Source: CAD feature listing. Evaluate the final solid. Frame: model axes, mm. Face numbers are marked on the shaded views. Coordinates: 2 decimals unless noted, no trailing zeros. Write each loop counter-clockwise with the first axis right and the second up, starting at its lowest first coordinate (ties: lowest second). Pieces come first, ordered by that corner, then holes. Notation, with made-up numbers: M 58.5,17.25 L 91.5,17.25 A32 cw 91.5,46.25 Z; hole C -23.5,-17.75 d6. An arc over 180 degrees is marked long. Write item = value, one per line. Start each with the question number.
1. Section query C-C (z = 4). Output: boundary loops of the cut face in (x, y), then the cut area to 3 significant figures.
2. Section query A-A (z = 11.5). Output: boundary loops of the cut face in (x, y), then the cut area to 3 significant figures.
3. Line query: line 1 along Y through (x, z) = (3.75, 12.5); line 2 along Z through (x, y) = (4.25, 1.75); line 3 along Y through (x, z) = (-6.5, -5). Output: solid intervals per line, ascending.
4. Pin query (flat end, axial travel): pin 1 Ø9 at (x, z) = (-2, 5) entering from -Y; pin 2 Ø4 at (x, y) = (4, -4) entering from +Z. Return the tip coordinate at first contact, or that it passes through.
5. Section query D-D (y = -2.5). Output: boundary loops of the cut face in (x, z).
6. Section query B-B (x = -2). Output: boundary loops of the cut face in (y, z), then the cut area to 3 significant figures.
7. Pull-direction query (Y, two-part tool) for the marked faces 1 and 2; classes: pulls with the +Y half, pulls with the -Y half, needs draft (parallel to the pull), parting line crosses it, or undercut.
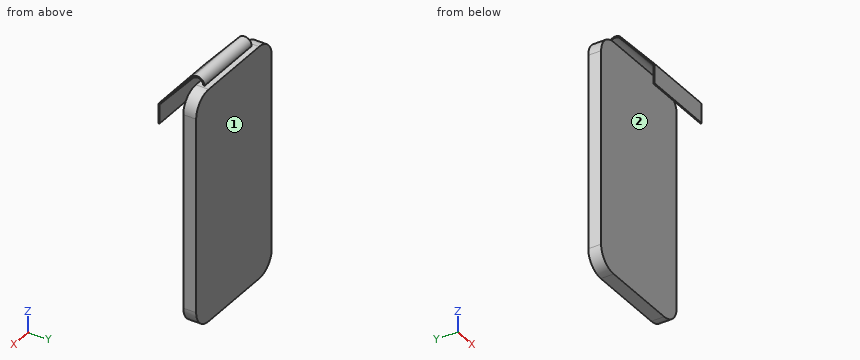
```python
from build123d import *

# Parameters (mm, degrees)
SKETCH_1_W      = 18.1
SKETCH_1_H      = 36.2
EXTRUDE_1_DEPTH = 2
FILLET_1_R      = 3
EXTRUDE_2_DEPTH = 5.65


with BuildPart() as part:
    # 草图1 → 凸台-拉伸1 (new body)
    with BuildSketch(Plane(origin=(0, 0, 0), x_dir=(1, 0, 0), z_dir=(0, 1, 0))):
        Rectangle(SKETCH_1_W, SKETCH_1_H)
    extrude(amount=EXTRUDE_1_DEPTH)

    # 圆角1
    fillet_1_edges = [part.edges().sort_by_distance(p)[0] for p in [
        (9.05, 1, 18.1),
        (-9.05, 1, 18.1),
        (-9.05, 1, -18.1),
        (9.05, 1, -18.1),
    ]]
    fillet(fillet_1_edges, radius=FILLET_1_R)

    # 草图2 → 凸台-拉伸2 (add, symmetric)
    with BuildSketch(Plane(origin=(0, 0, 0), x_dir=(0, 0, -1), z_dir=(1, 0, 0))):
        with BuildLine():
            Line((-18.821174134, -0.830606928), (-12.752189981, -6.1))
            Line((-12.752189981, -6.1), (-9.714835193, -6.1))
            Line((-9.714835193, -6.1), (-9.714835193, -5.9))
            Line((-9.714835193, -5.9), (-12.677480404, -5.9))
            Line((-12.677480404, -5.9), (-18.690051564, -0.679587486))
            ThreePointArc((-18.690051564, -0.679587486), (-18.943098078, 0.314937504), (-18.1, 0.9))
            Line((-18.1, 0.9), (-18.1, 1.1))
            ThreePointArc((-18.1, 1.1), (-19.130453206, 0.384923615), (-18.821174134, -0.830606928))
        make_face()
    extrude(amount=EXTRUDE_2_DEPTH, both=True)


solid = part.part
```
Results are:
q1.outline = M -9.05,0 L 9.05,0 L 9.05,2 L -9.05,2 Z
q1.area = 36.2 mm^2
q2.outline = M -9.05,0 L 9.05,0 L 9.05,2 L -9.05,2 Z; M -5.65,-6.1 L 5.65,-6.1 L 5.65,-5.9 L -5.65,-5.9 Z
q2.area = 38.5 mm^2
q3.line_1 = -6.1 to -5.9, 0 to 2
q3.line_2 = -18.1 to 18.1
q3.line_3 = 0 to 2
q4.pin_1 = 0
q4.pin_2 = 17.47
q5.outline = M -5.65,16.59 L 5.65,16.59 L 5.65,16.9 L -5.65,16.9 Z
q6.outline = M -6.1,9.71 L -5.9,9.71 L -5.9,12.68 L -0.68,18.69 A0.9 cw 0.9,18.1 L 0,18.1 L 0,-18.1 L 2,-18.1 L 2,18.1 L 1.1,18.1 A1.1 ccw -0.83,18.82 L -6.1,12.75 Z
q6.area = 75.1 mm^2
q7.face_1 = pulls with the +Y half
q7.face_2 = undercut
